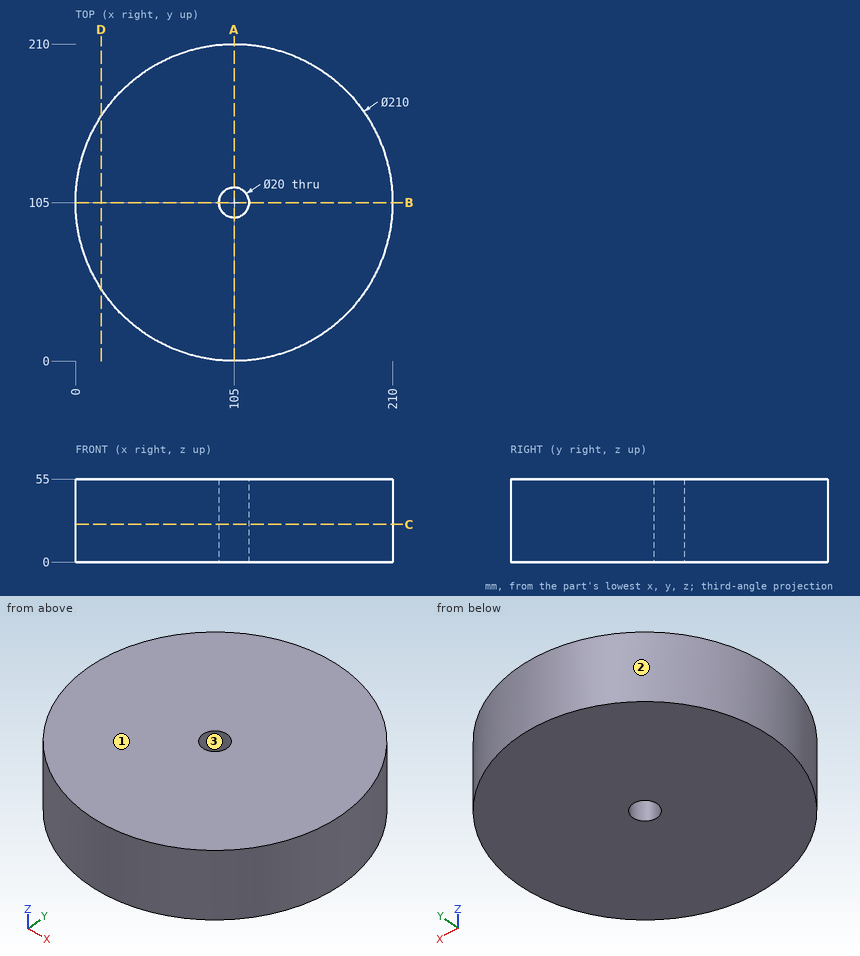
For this review, use the dimensioned drawing (mm, ordinates from the lowest corner) and the shaded views. Coordinates: 2 decimals unless noted, no trailing zeros. Order: outer loops, then holes, each group sorted by start corner. A loop starts at its lowest first (then second) coordinate and runs counter-clockwise, first axis right, second up. Notation, with made-up numbers: (57.25, 53) -> (70.25, 53) arc R13 cw to (70.25, 77) -> close; hole circle Ø10 at (8, 36.25). An arc over 180 degrees is marked (long way). One line per item, written item: value. Start each with the question number.
Q1. Mouldability with a two-part tool opening along Y and no side actions: class the marked faces 1, 2 and 3 as pulls with the +Y half, pulls with the -Y half, needs draft (parallel to the pull), parting line crosses it, or undercut.
Q2. Take a section at D-D, the plane x = 17. State the section outline as (y, z) points, then the cut area to 3 significant figures.
Q3. For probe 1 along Y at (x, z) = (105, 26); probe 2 along Y at (x, z) = (111, 15.5); probe 3 along Y at (x, z) = (15.5, 30), list the stretches that pass through material, from the lowest coordinate up.
Q4. Insertion check: pin 1 Ø1 at (x, z) = (66.5, 7.5) entering from +Y; pin 2 Ø1.5 at (y, z) = (113.5, 9.5) entering from +X; pin 3 Ø10 at (y, z) = (69.5, 6.5) entering from +X. Each pin has a flat end and moves straight along its axis. Give the tip position at first contact, or say it passes through.
Q5. Take a section at A-A, the plane x = 105. State the section outline as (y, z) points, then the cut area to 4 significant figures.
Q6. Take a section at C-C, the plane z = 25. State the section outline as (x, y) points.
Values follow:
1. face 1: needs draft
1. face 2: parting line crosses it
1. face 3: undercut
2. outline: (47.72, 0) -> (162.28, 0) -> (162.28, 55) -> (47.72, 55) -> close
2. area: 6,300 mm2
3. probe 1: y = 0 to 95, 115 to 210
3. probe 2: y = 0.17 to 97, 113 to 209.83
3. probe 3: y = 50.09 to 159.91
4. pin 1: stops at y = 202.88
4. pin 2: stops at x = 209.71
4. pin 3: stops at x = 205.47
5. outline: (0, 0) -> (95, 0) -> (95, 55) -> (0, 55) -> close; (115, 0) -> (210, 0) -> (210, 55) -> (115, 55) -> close
5. area: 10,450 mm2
6. outline: circle Ø210 at (105, 105); hole circle Ø20 at (105, 105)
